```python
from build123d import *

# Parameters (mm, degrees)
SKETCH_1_W               = 50
SKETCH_1_H               = 40
EXTRUDE_1_DEPTH          = 40
CUT_EXTRUDE_1_DEPTH      = 76.498344353
CUT_EXTRUDE_1_DEPTH_BACK = 76.498344353
SKETCH_4_W               = 5
SKETCH_4_H               = 4
CUT_EXTRUDE_3_DEPTH      = 76.498344353
CUT_EXTRUDE_3_DEPTH_BACK = 76.498344353
CUT_EXTRUDE_4_DEPTH      = 76.498344353
CUT_EXTRUDE_4_DEPTH_BACK = 76.498344353
SKETCH_6_W               = 41
SKETCH_6_H               = 5
CUT_EXTRUDE_5_DEPTH      = 76.498344353
CUT_EXTRUDE_5_DEPTH_BACK = 7
CUT_EXTRUDE_6_DEPTH      = 76.498344353
CUT_EXTRUDE_6_DEPTH_BACK = 10
CUT_EXTRUDE_7_DEPTH      = 76.498344353
CUT_EXTRUDE_7_DEPTH_BACK = 9
CUT_EXTRUDE_8_DEPTH      = 76.498344353
CUT_EXTRUDE_8_DEPTH_BACK = 9
CUT_EXTRUDE_9_DEPTH      = 76.498344353
CUT_EXTRUDE_9_DEPTH_BACK = 9
SKETCH_15_W              = 11
SKETCH_15_H              = 7


with BuildPart() as part:
    # Эскиз1 → Бобышка-Вытянуть1 (new body)
    with BuildSketch(Plane(origin=(0, 0, 0), x_dir=(1, 0, 0), z_dir=(0, 1, 0))):
        with Locations((25, 20)):
            Rectangle(SKETCH_1_W, SKETCH_1_H)
    extrude(amount=EXTRUDE_1_DEPTH)

    # Эскиз4 → Вырез-Вытянуть1 (cut, two sides: drawn at the far end of the back side and taken through both)
    with BuildSketch(Plane.XY.offset(-CUT_EXTRUDE_1_DEPTH_BACK)):
        with Locations((22.5, 2)):
            Rectangle(SKETCH_4_W, SKETCH_4_H)
        with Locations((27.5, 2)):
            Rectangle(SKETCH_4_W, SKETCH_4_H)
    extrude(amount=CUT_EXTRUDE_1_DEPTH + CUT_EXTRUDE_1_DEPTH_BACK, mode=Mode.SUBTRACT)

    # Эскиз5 → Вырез-Вытянуть3 (cut, two sides: drawn at the far end of the back side and taken through both)
    with BuildSketch(Plane.ZY.offset(-CUT_EXTRUDE_3_DEPTH_BACK)):
        Polygon((-20, 4), (-26.721648091, 0), (-13.278351909, 0), align=None)
    extrude(amount=CUT_EXTRUDE_3_DEPTH + CUT_EXTRUDE_3_DEPTH_BACK, mode=Mode.SUBTRACT)

    # Эскиз6 → Вырез-Вытянуть4 (cut, two sides: drawn at the far end of the back side and taken through both)
    with BuildSketch(Plane.XY.offset(-CUT_EXTRUDE_4_DEPTH_BACK)):
        with Locations((29.5, 37.5)):
            Rectangle(SKETCH_6_W, SKETCH_6_H)
    extrude(amount=CUT_EXTRUDE_4_DEPTH + CUT_EXTRUDE_4_DEPTH_BACK, mode=Mode.SUBTRACT)

    # Эскиз8 → Вырез-Вытянуть5 (cut, two sides: drawn at the far end of the back side and taken through both)
    with BuildSketch(Plane.XY.offset(-CUT_EXTRUDE_5_DEPTH_BACK)):
        with BuildLine():
            ThreePointArc((0, 3), (9.466087362, 17.921086779), (14, 35))
            Line((14, 35), (9, 35))
            Line((9, 35), (9, 40))
            Line((9, 40), (0, 40))
            Line((0, 40), (0, 3))
        make_face()
    extrude(amount=CUT_EXTRUDE_5_DEPTH + CUT_EXTRUDE_5_DEPTH_BACK, mode=Mode.SUBTRACT)

    # Эскиз9 → Вырез-Вытянуть6 (cut, two sides: drawn at the far end of the back side and taken through both)
    with BuildSketch(Plane(origin=(50, 0, 0), x_dir=(0, 0, -1), z_dir=(1, 0, 0)).offset(-CUT_EXTRUDE_6_DEPTH_BACK)):
        Polygon((0, 35), (0, 3), (7, 35), align=None)
    extrude(amount=CUT_EXTRUDE_6_DEPTH + CUT_EXTRUDE_6_DEPTH_BACK, mode=Mode.SUBTRACT)

    # Эскиз11 → Вырез-Вытянуть7 (cut, two sides: drawn at the far end of the back side and taken through both)
    with BuildSketch(Plane.ZY.offset(-CUT_EXTRUDE_7_DEPTH_BACK)):
        Polygon((-150, 22), (-40, 22), (-30, 22), (-30, 40), (-30, 150), (-190.498184911, 300.467048354), (-310.498184911, 172.467048354), align=None)
    extrude(amount=CUT_EXTRUDE_7_DEPTH + CUT_EXTRUDE_7_DEPTH_BACK, mode=Mode.SUBTRACT)

    # Эскиз14 → Вырез-Вытянуть8 (cut, two sides: drawn at the far end of the back side and taken through both)
    with BuildSketch(Plane.ZY.offset(-CUT_EXTRUDE_8_DEPTH_BACK)):
        Polygon((-7, 40), (-18.5, 40), (-7, 37), align=None)
    extrude(amount=CUT_EXTRUDE_8_DEPTH + CUT_EXTRUDE_8_DEPTH_BACK, mode=Mode.SUBTRACT)

    # Эскиз15 → Вырез-Вытянуть9 (cut, two sides: drawn at the far end of the back side and taken through both)
    with BuildSketch(Plane(origin=(0, 0, -40), x_dir=(-1, 0, 0), z_dir=(0, 0, -1)).offset(-CUT_EXTRUDE_9_DEPTH_BACK)):
        with Locations((-44.5, 31.5)):
            Rectangle(SKETCH_15_W, SKETCH_15_H)
    extrude(amount=CUT_EXTRUDE_9_DEPTH + CUT_EXTRUDE_9_DEPTH_BACK, mode=Mode.SUBTRACT)


solid = part.part
```
The listing builds one solid part. Answer for the finished solid, in the listing's coordinates (mm). A direction names the side the tool comes from. Round coordinates to 2 decimals unless told otherwise and drop trailing zeros. Loops run counter-clockwise (first coordinate to the right, second up) from the corner with the lowest first, then second, coordinate; pieces in that order, holes last.
Q1. Section C-C, the plane z = -4.5 is taken. Determine the outline of the cut face in (x, y).
Q2. Section B-B, the plane y = 2 is taken. Determine the outline of the cut face in (x, z), then the cut area to 3 significant figures.
Q3. For a pull along Z with two mould halves and no side action, classify faces 6 (the face through (10.14, 1.97, -16.59)), 7 (the face through (45, 32, -31)), 8 (the face through (9, 37, -19)) as released by +Z, released by -Z, zero draft, split by the parting line, or undercut.
Q4. Section D-D, the plane y = 23 is taken. Determine the outline of the cut face in (x, z) (3 decimals).
Q5. Find the intervals of material crossed by line 1 (X direction, y = 2, z = -24); line 2 (Y direction, x = 26, z = -8); line 3 (Z direction, x = 38.5, y = 3.5), in increasing order.
Q6. Section A-A, the plane x = 43.5 is taken. Determine the outline of the cut face in (y, z).
Q7. Given pin 1 Ø3.5 at (y, z) = (32, -36) entering from +X; pin 2 Ø4 at (y, z) = (37.5, -16) entering from +X; pin 3 Ø2 at (x, y) = (46, 32.5) entering from -Z, each flat-ended and moving along its own axis, determine where each tip first touches the part or whether it passes through.
Q8. Which of the six approach directions +Z, -Z, +X, -X, +Y, -Y give full straight-line access (tool end or side, diameter ignored) to faces 1 (the face through (5, 31, -30)), 2 (the face through (20, 2, -8)), 3 (the face through (5, 24, -7)), 4 (the face through (44.93, 18.78, -3.45)), 5 (the face through (10.14, 2.03, -23.31))?
Completed:
1. outline: (0, 0) - (20, 0) - (20, 4) - (30, 4) - (30, 0) - (50, 0) - (50, 23.57) - (40, 23.57) - (40, 35) - (14, 35) arc R58 cw to (0, 3) - close
2. outline: (0, -40) - (20, -40) - (20, -23.36) - (0, -23.36) - close; (0, -16.64) - (20, -16.64) - (20, 0) - (0, 0) - close; (30, -40) - (50, -40) - (50, -23.36) - (30, -23.36) - close; (30, -16.64) - (50, -16.64) - (50, 0) - (30, 0) - close
2. area: 1,330 mm2
3. face 6: undercut
3. face 7: released by -Z
3. face 8: zero draft
4. outline: (0, -30) - (9, -30) - (9, -40) - (50, -40) - (50, -4.375) - (40, -4.375) - (40, 0) - (11.41, 0) - (11.41, -7) - (0, -7) - close
5. line 1: x = 0 to 20, 30 to 50
5. line 2: y = 4 to 35
5. line 3: z = -40 to -20.84, -19.16 to 0
6. outline: (0, -40) - (28, -40) - (28, -31) - (35, -31) - (35, -7) - (3, 0) - (0, 0) - (0, -13.28) - (4, -20) - (0, -26.72) - close
7. pin 1: stops at x = 39
7. pin 2: stops at x = 9
7. pin 3: stops at z = -31
8. face 1: -Z, -X, +Y
8. face 2: +Z, -Z, -Y
8. face 3: +Z, -X, +Y
8. face 4: +Z, +X, +Y
8. face 5: +X, -X, -Y
